Check sheet for the drawn part. Datum: minimum x, y, z corner. Units: mm. A direction names the side the tool comes from. Give positions to 0.01 mm unless a question says otherwise; leave off trailing zeros. Order: outer loops, then holes, each group sorted by start corner. A loop starts at its lowest first (then second) coordinate and runs counter-clockwise, first axis right, second up.
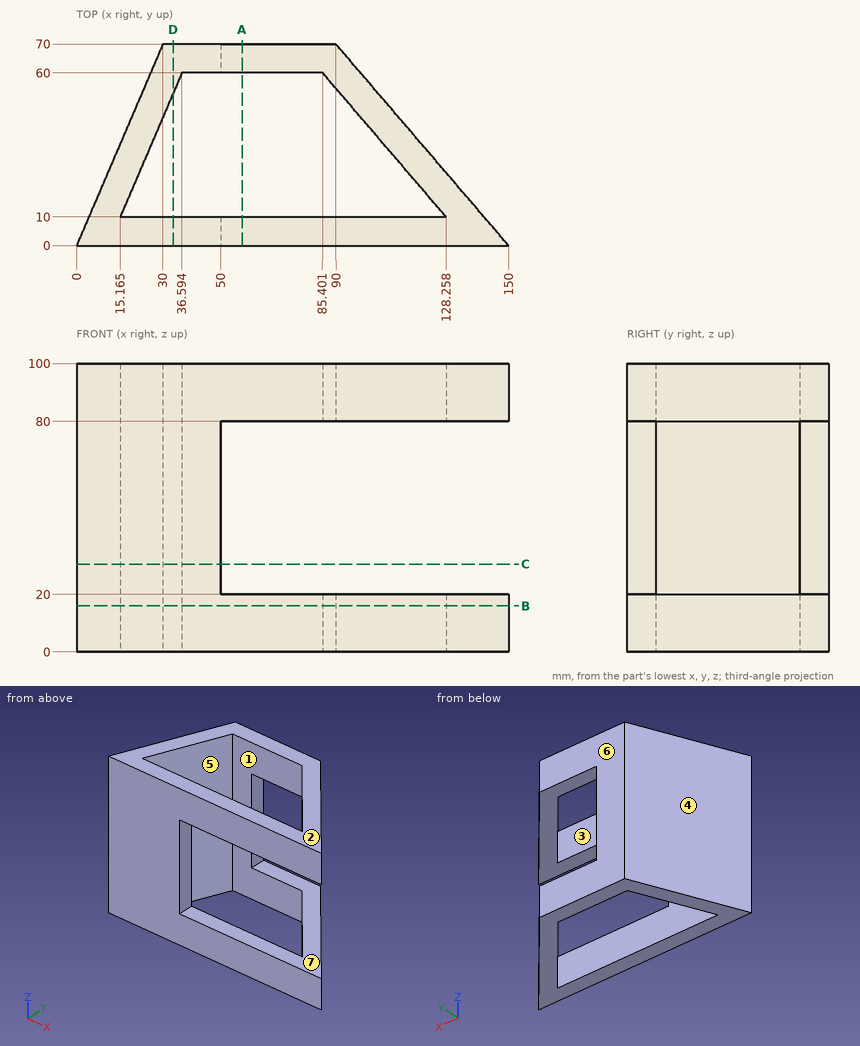
(1) Section check A-A, the plane x = 57.5. Enter the section's corners in (y, z), then the cut area to 3 significant figures.
Solved:
outline: (0, 0) - (10, 0) - (10, 20) - (0, 20) - close; (0, 80) - (10, 80) - (10, 100) - (0, 100) - close; (60, 0) - (70, 0) - (70, 20) - (60, 20) - close; (60, 80) - (70, 80) - (70, 100) - (60, 100) - close
area: 800 mm2
(2) Section check C-C, the plane z = 30.5. Enter the section's corners in (x, y) (1 decimal).
Solved:
outline: (0, 0) - (50, 0) - (50, 10) - (15.2, 10) - (36.6, 60) - (50, 60) - (50, 70) - (30, 70) - close
(3) Section check D-D, the plane x = 33.5. Enter the section's corners in (y, z), then the cut area to 3 significant figures.
Solved:
outline: (0, 0) - (10, 0) - (10, 100) - (0, 100) - close; (52.78, 0) - (70, 0) - (70, 100) - (52.78, 100) - close
area: 2,720 mm2
(4) Set-up check for the marked faces 5, 6 and 7: record each of +Z, -Z, +X, -X, +Y, -Y from which the full face is reachable in a straight line by a thin tool's end or side.
Solved:
face 5: +Z, -Z
face 6: +Z, -Z, +X, -X, +Y
face 7: +X, +Y, -Y
(5) Release check for a two-part mould opening along X. For the marked faces 1, 2, 3 and 4 record: pulls with the +X half, pulls with the -X half, needs draft (parallel to the pull), parting line crosses it, or undercut.
Solved:
face 1: undercut
face 2: needs draft
face 3: undercut
face 4: pulls with the -X half
(6) Go/stop test with flat-tipped pins: pin 1 (8 mm diameter, centred on y = 60.5, z = 13.5, fed in from +X); pin 2 (3 mm diameter, centred on y = 19.5, z = 87.5, fed in from +X); pin 3 (6 mm diameter, centred on y = 18.5, z = 43, fed in from +X); pin 4 (10 mm diameter, centred on x = 58, y = 57, fed in from -Z). Record where each tip stops, or that it passes through.
Solved:
pin 1: stops at x = 101.57
pin 2: stops at x = 134.57
pin 3: stops at x = 20.09
pin 4: stops at z = 0
(7) Scan lines: line 1 (Z direction, x = 75, y = 65); line 2 (Y direction, x = 46.5, z = 15.5); line 3 (X direction, y = 24, z = 13.5) (1 decimal). Record each from-to range of solid material in increasing order.
Solved:
line 1: z = 0 to 20, 80 to 100
line 2: y = 0 to 10, 60 to 70
line 3: x = 10.3 to 21.2, 116.3 to 129.4
(8) Section check B-B, the plane z = 16. Enter the section's corners in (x, y) (1 decimal), then the cut area to 3 significant figures.
Solved:
outline: (0, 0) - (150, 0) - (90, 70) - (30, 70) - close; hole (15.2, 10) - (128.3, 10) - (85.4, 60) - (36.6, 60) - close
area: 3,300 mm2
